Work out the finished part from the listing and answer in its coordinate system (mm). Face numbers are marked on the shaded views. Coordinates: 2 decimals unless noted, no trailing zeros. Order: outer loops, then holes, each group sorted by start corner. A loop starts at its lowest first (then second) coordinate and runs counter-clockwise, first axis right, second up.
1. Find the intervals of material crossed by probe 1 along Z at (x, y) = (0, 93.5); probe 2 along X at (y, z) = (88.5, 0.25); probe 3 along X at (y, z) = (120.5, -1.75), in increasing order.
2. The part is cut by section A-A, the plane y = 75. Give the vertices of the cut face in (x, z), then the cut area to 3 significant figures.
3. Flat-ended cylindrical pins translate along their axes: pin 1 Ø4 at (x, z) = (0.5, 0) entering from +Y; pin 2 Ø4 at (y, z) = (85, 2) entering from +X; pin 3 Ø1.5 at (y, z) = (39, -3) entering from -X. Find the tip coordinate at first contact, or state that the pin passes through.
4. Determine the mould class of the marked faces 1 and 2 for opening direction Y: +Y half, -Y half, draft (parallel to the pull), parting line (faces both ways), or undercut.
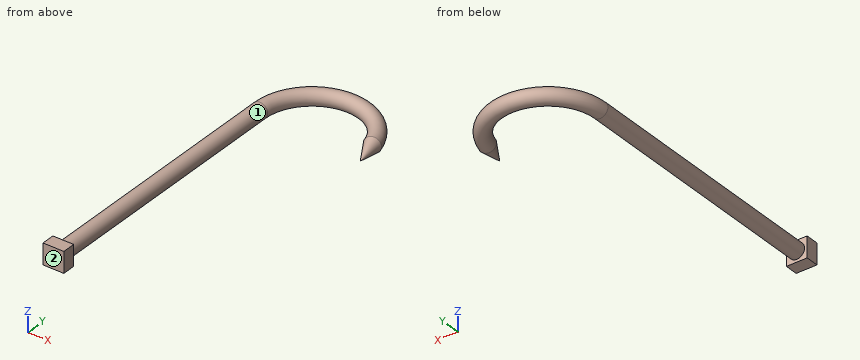
```python
from build123d import *

# Parameters (mm, degrees)
SKETCH1_W           = 8
SKETCH1_H           = 8
BOSS_EXTRUDE1_DEPTH = 5
SKETCH3_R           = 3
CHAMFER1_SIZE2      = 3
CHAMFER1_SIZE       = 10


with BuildPart() as part:
    # Sketch1 → Boss-Extrude1 (new body)
    with BuildSketch(Plane(origin=(0, 0, 0), x_dir=(1, 0, 0), z_dir=(0, 1, 0))):
        Rectangle(SKETCH1_W, SKETCH1_H)
    extrude(amount=BOSS_EXTRUDE1_DEPTH)

    # Sweep1: sweep along a path in Sketch2
    with BuildLine(Plane.XY) as sweep1_path:
        Line((0, 5), (0, 105))
        ThreePointArc((0, 105), (17.389476156, 124.828897227), (39.318516526, 110.176380902))
        Line((39.318516526, 110.176380902), (41.906706977, 100.517122639))
    # Sketch3 → Sweep1 (sweep)
    with BuildSketch(Plane(origin=(0, 5, 0), x_dir=(1, 0, 0), z_dir=(0, 1, 0))):
        Circle(SKETCH3_R)
    sweep(path=sweep1_path.line)

    # Chamfer1
    chamfer1_edges = [part.edges().sort_by_distance(p)[0] for p in [
        (44.804484456, 101.293579774, 0),
    ]]
    chamfer1_side = [part.faces().sort_by_distance(p)[0] for p in [
        (44.788955313, 101.351535324, 0),
    ]]
    chamfer(chamfer1_edges, length=CHAMFER1_SIZE - 0.0001, length2=CHAMFER1_SIZE2 - 0.0001, reference=chamfer1_side[0])  # a hair under: the kernel refuses the full size


solid = part.part
```
Geometry says:
1. probe 1: z = -3 to 3
1. probe 2: x = -2.99 to 2.99
1. probe 3: x = 3.78 to 11.74, 28.26 to 36.22
2. outline: circle Ø6 at (0, 0)
2. area: 28.3 mm2
3. pin 1: stops at y = 119.92
3. pin 2: stops at x = 3
3. pin 3: stops at x = -1.98
4. face 1: undercut
4. face 2: -Y half
